Build history of the part. All positions in model axes, mm. A direction names the side the tool comes from. Round coordinates to 2 decimals unless told otherwise and drop trailing zeros. Order: outer loops, then holes, each group sorted by start corner. A loop starts at its lowest first (then second) coordinate and runs counter-clockwise, first axis right, second up. Notation, with made-up numbers: M 39,39 L 43,39 A33 ccw 43,71 Z; hole C 36.25,43 d4. An arc over 180 degrees is marked long. One line per item, written item: value. Start each with the question number.
Item 1: Probe L1, parallel to Y at x = 1.5, z = -59.5; L2, parallel to Z at x = 170, y = -3.5. List the from-to ranges inside material, lowest first.
Item 2: Pin check, flat tips, straight feed: pin 1 (2 mm diameter, centred on x = 160.5, y = -4, fed in from +Z); pin 2 (2 mm diameter, centred on y = -4.5, z = -60.5, fed in from +X); pin 3 (1.2 mm diameter, centred on y = -3.5, z = -51.5, fed in from -X); pin 4 (2 mm diameter, centred on y = -3, z = 77.5, fed in from -X). Stop position of each tip, or through.
Item 3: Tool access for faces 1 (the flat face through (161, -2.5, -52)), 2 (the flat face through (11, -2.5, 75)), 3 (the flat face through (11, -2.5, -52)): list every direction of +Z, -Z, +X, -X, +Y, -Y with a clear straight run to the whole face (end or side of a thin tool).
Item 4: Band-saw the part on B-B, the plane x = 0.5. Write the cut outline in (y, z).
Item 5: Band-saw the part on A-A, the plane z = 64.5. Write the cut outline in (x, y), then the cut area to 3 significant figures.
Autodesk Inventor part; units mm, degrees
ref_plane "YZ Plane" through (0, 0, 0) normal (1, 0, 0) x (0, 1, 0)
ref_plane "XZ Plane" through (0, 0, 0) normal (0, 1, 0) x (-1, 0, 0)
ref_plane "XY Plane" through (0, 0, 0) normal (0, 0, 1) x (1, 0, 0)
sketch "Sketch1" plane through (0, 0, 0) normal (0, 1, 0) x (-1, 0, 0)
  line L0 (13.84, 90.8) -> (-186.16, 90.8)
  line L1 (-186.16, 90.8) -> (-186.16, -69.2)
  line L2 (-186.16, -69.2) -> (13.84, -69.2)
  line L3 (13.84, -69.2) -> (13.84, 90.8)
  point P0 (0, 0)
  dimension "d0" = 160
  dimension "d1" = 200
extrude "Extrusion1" add sketch "Sketch1" along normal blind 11
sketch "Sketch2" plane through (186.16, 0, 90.8) normal (1, 0, 0) x (0, 0, -1)
  line L0 (0, 0) -> (0, 11)
  line L1 (0, 0) -> (-12, 0)
  line L2 (-12, 0) -> (-12, 60)
  line L3 (-12, 60) -> (0, 60)
  line L4 (0, 60) -> (0, 0)
  line L5 (160, 0) -> (160, 11)
  line L6 (160, 0) -> (172, 0)
  line L7 (172, 0) -> (172, 60)
  line L8 (172, 60) -> (160, 60)
  line L9 (160, 60) -> (160, 0)
  point P0 (90.8, 0)
  point P1 (0, 11)
  dimension "d4" = 60
  dimension "d5" = 60
  dimension "d6" = 12
  dimension "d17" = 12
extrude "Extrusion2" add sketch "Sketch2" against normal up to surface (200 mm away)
sketch "Sketch3" plane through (0, 0, 0) normal (0, -1, 0) x (1, 0, 0)
  line L0 (186.16, 102.8) -> (186.16, -81.2)
  line L1 (186.16, 102.8) -> (-13.84, 102.8)
  line L2 (-13.84, -81.2) -> (-13.84, 102.8)
  line L3 (186.16, -81.2) -> (-13.84, -81.2)
  point P0 (0, 0)
extrude "Extrusion3" add sketch "Sketch3" along normal blind 5
sketch "Sketch7" plane through (0, 11, 0) normal (0, 1, 0) x (1, 0, 0)
  line L0 (186.16, -90.8) -> (-13.84, -90.8)
  line L1 (36.16, -90.8) -> (136.16, -90.8)
  line L2 (136.16, -90.8) -> (136.16, -65.8)
  line L3 (136.16, -65.8) -> (36.16, -65.8)
  line L4 (36.16, -65.8) -> (36.16, -90.8)
  line L5 (186.16, 69.2) -> (-13.84, 69.2)
  line L6 (36.16, 69.2) -> (136.16, 69.2)
  line L7 (136.16, 69.2) -> (136.16, 44.2)
  line L8 (136.16, 44.2) -> (36.16, 44.2)
  line L9 (36.16, 44.2) -> (36.16, 69.2)
  line L10 (-13.84, 69.2) -> (-13.84, -90.8)
  line L11 (186.16, -90.8) -> (186.16, 69.2)
  point P0 (0, 0)
  point P1 (136.16, 56.7)
  dimension "d18" = 25
  dimension "d19" = 25
  dimension "d20" = 50
  dimension "d21" = 50
  dimension "d22" = 50
  dimension "d23" = 50
extrude "Extrusion6" add sketch "Sketch7" along normal blind 10 contours L0 L4 L3 L2 | L7 L8 L9 L5
fillet "Fillet1" radius 4 4 edges at (36.16, 16, -69.2) (36.16, 16, 90.8) (136.16, 16, -69.2) (136.16, 16, 90.8)
fillet "Fillet2" radius 10 4 edges at (138.16, 21, -69.2) (34.16, 21, -69.2) (34.16, 21, 90.8) (138.16, 21, 90.8)
sketch "Sketch8" plane through (-13.84, 11, 90.8) normal (-1, 0, 0) x (0, 0, 1)
  line L0 (-160, 0) -> (0, 0)
  line L1 (0, 0) -> (0, -19)
  line L2 (0, -19) -> (-160, -19)
  line L3 (-160, -19) -> (-160, 0)
  line L4 (-172, 49) -> (12, 49)
  line L5 (12, 49) -> (12, -16)
  line L6 (12, -16) -> (-172, -16)
  line L7 (-172, -16) -> (-172, 49)
  point P0 (-90.8, -11)
  point P1 (0, -16)
  point P2 (-160, -16)
extrude "Extrusion7" cut sketch "Sketch8" against normal blind 1000 contours L3 L6 L7 L4 L5 L1 L0
sketch "Sketch10" plane through (0, -5, 0) normal (0, -1, 0) x (1, 0, 0)
  line L0 (186.16, -69.2) -> (-13.84, -69.2)
  line L1 (-13.84, -69.2) -> (36.16, -69.2)
  line L2 (36.16, -69.2) -> (36.16, -36.2)
  line L3 (36.16, -36.2) -> (-13.84, -36.2)
  line L4 (-13.84, -36.2) -> (-13.84, -69.2)
  line L5 (186.16, -69.2) -> (136.16, -69.2)
  line L6 (136.16, -69.2) -> (136.16, -36.2)
  line L7 (136.16, -36.2) -> (186.16, -36.2)
  line L8 (186.16, -36.2) -> (186.16, -69.2)
  line L9 (186.16, 90.8) -> (136.16, 90.8)
  line L10 (136.16, 90.8) -> (136.16, 57.8)
  line L11 (136.16, 57.8) -> (186.16, 57.8)
  line L12 (186.16, 57.8) -> (186.16, 90.8)
  line L13 (-13.84, 90.8) -> (36.16, 90.8)
  line L14 (36.16, 90.8) -> (36.16, 57.8)
  line L15 (36.16, 57.8) -> (-13.84, 57.8)
  line L16 (-13.84, 57.8) -> (-13.84, 90.8)
  line L17 (186.16, 90.8) -> (-13.84, 90.8)
  point P0 (0, 0)
  dimension "d30" = 50
  dimension "d31" = 50
  dimension "d32" = 50
  dimension "d33" = 50
  dimension "d34" = 33
  dimension "d35" = 33
  dimension "d36" = 0
extrude "Extrusion8" cut sketch "Sketch10" against normal blind 2.5
properties part number "Y_karetka" material "Aluminum 6061"
Output:
1. L1: y = -2.5 to 11
1. L2: z = -36.2 to 57.8
2. pin 1: stops at z = 57.8
2. pin 2: stops at x = 136.16
2. pin 3: stops at x = 36.16
2. pin 4: stops at x = -13.84
3. face 1: -Z, +X, -Y
3. face 2: +Z, -X, -Y
3. face 3: -Z, -X, -Y
4. outline: M -5,-36.2 L -2.5,-36.2 L -2.5,-69.2 L 11,-69.2 L 11,90.8 L -2.5,90.8 L -2.5,57.8 L -5,57.8 Z
5. outline: M -13.84,-2.5 L 36.16,-2.5 L 36.16,-5 L 136.16,-5 L 136.16,-2.5 L 186.16,-2.5 L 186.16,11 L -13.84,11 Z
5. area: 2,950 mm²
